The listing builds one solid part. Answer for the finished solid, in the listing's coordinates (mm). Give positions to 0.01 mm unless a question says otherwise; leave off trailing zeros. Order: outer loops, then holes, each group sorted by start corner. A loop starts at its lowest first (then second) coordinate and runs counter-clockwise, first axis right, second up. Notation, with made-up numbers: (-26.75, -30) - (21.25, -30) arc R36 cw to (21.25, 7) - close; hole circle Ø8 at (-7.5, 69). An arc over 180 degrees is marked (long way). Answer as a JSON object with one key per item and string values. Group by question number.
Q1. A cutting plane is placed at C-C, the plane x = 35.5. Give the vertices of the cut face in (y, z), and give its area (3 significant figures).
Q2. A cutting plane is placed at D-D, the plane z = 20. Give the vertices of the cut face in (x, y), and give its area (3 significant figures).
Q3. A cutting plane is placed at B-B, the plane x = 5. Give the vertices of the cut face in (y, z).
Q4. Given pin 1 (18 mm diameter, centred on x = 16.42, z = 30, fed in from +Y), flat-ended and moving along its own axis, determine where the tip first touches the part or whether it passes through.
Q5. A cutting plane is placed at A-A, the plane z = 30. Give the vertices of the cut face in (x, y).
Q6. Consider line 1 (X direction, y = 3.9, z = 30); line 2 (X direction, y = 3.4, z = 55); line 3 (Z direction, x = 5.5, y = 4). Determine where each line is inside the solid, lowest interval first.
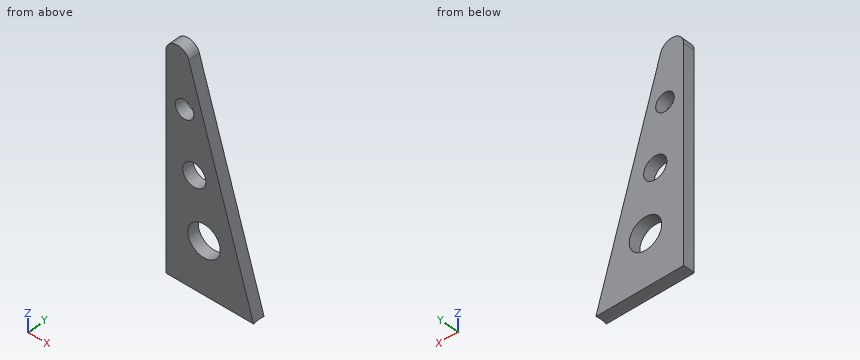
from build123d import *

# Parameters (mm, degrees)
SKETCH1_R           = 4
SKETCH1_R_2         = 5
SKETCH1_R_3         = 7
BOSS_EXTRUDE1_DEPTH = 5
SKETCH2_R           = 12.7
CUT_EXTRUDE1_DEPTH  = 50


with BuildPart() as part:
    # Sketch1 → Boss-Extrude1 (new body)
    with BuildSketch(Plane(origin=(0, 0, 0), x_dir=(1, 0, 0), z_dir=(0, 1, 0))):
        with BuildLine():
            Line((0, 0), (0, -100))
            ThreePointArc((0, -100), (4.326195296, -105), (9.896144859, -101.437468934))
            Line((9.896144859, -101.437468934), (40, 0))
            Line((40, 0), (0, 0))
        make_face()
        with Locations(Location((8.0237285, -80, 0), (0, 0, 270))):
            Circle(SKETCH1_R, mode=Mode.SUBTRACT)
        with Locations(Location((12.222443443, -55, 0), (0, 0, 270))):
            Circle(SKETCH1_R_2, mode=Mode.SUBTRACT)
        with Locations(Location((16.421158385, -30, 0), (0, 0, 270))):
            Circle(SKETCH1_R_3, mode=Mode.SUBTRACT)
    extrude(amount=BOSS_EXTRUDE1_DEPTH)

    # Sketch2 → Cut-Extrude1 (cut)
    with BuildSketch(Plane.ZY):
        with Locations((-5, 2.5)):
            Circle(SKETCH2_R)
    extrude(amount=-CUT_EXTRUDE1_DEPTH, mode=Mode.SUBTRACT)


solid = part.part
Reply:
{
 "1": {"outline": "(0, 7.45) arc R12.7 cw to (5, 7.45) - (5, 15.16) - (0, 15.16) - close", "area": "37.7 mm^2"},
 "2": {"outline": "(0, 0) - (34.06, 0) - (34.06, 5) - (0, 5) - close", "area": "170 mm^2"},
 "3": {"outline": "(0, 7.45) arc R12.7 cw to (5, 7.45) - (5, 77.38) - (0, 77.38) - close; (0, 82.62) - (5, 82.62) - (5, 105.05) - (0, 105.05) - close"},
 "4": {"pin 1": "stops at y = 5"},
 "5": {"outline": "(0, 0) - (9.42, 0) - (9.42, 5) - (0, 5) - close; (23.42, 0) - (31.1, 0) - (31.1, 5) - (23.42, 5) - close"},
 "6": {"line 1": "x = 0 to 9.42, 23.42 to 31.1", "line 2": "x = 0 to 7.22, 17.22 to 23.68", "line 3": "z = 7.61 to 76.9, 83.1 to 105.03"}
}
